Geometry check sheet. Reference: the model listing, model coordinates, mm. A direction names the side the tool comes from. Round coordinates to 2 decimals unless told otherwise and drop trailing zeros. Order: outer loops, then holes, each group sorted by start corner. A loop starts at its lowest first (then second) coordinate and runs counter-clockwise, first axis right, second up. Notation, with made-up numbers: (43, -4) - (81, -4) arc R14 ccw to (81, 6) - close; hole circle Ø6 at (-16, 6.25). An arc over 180 degrees is marked (long way). One line per question, with ' | ' between items. Start each with the question number.
Q1. Sectioned sample at C-C, the plane x = 0. Give the number of separate pieces and of enclosed holes in the cut face, then the cut area to 3 significant figures.
Q2. Sectioned sample at A-A, the plane x = -30.5. Enter the section's corners in (y, z), then the cut area to 3 significant figures.
Q3. Material ranges on line 1 along Z through (x, y) = (9, 5); line 2 along Z through (x, y) = (-7, 34); line 3 along Y through (x, z) = (-33, -41.5), recorded low to high.
Q4. Gauge pin test, flat ends, axial feed: P1, Ø2, axis at x = -19.5, y = -16, coming from the +Z side; P2, Ø2, axis at y = -15.5, z = -18, coming from the +X side; P3, Ø5, axis at x = 23, y = 26.5, coming from the +Z side; P4, Ø1.5, axis at x = -31.5, z = -38.5, coming from the +Y side. Record the tip position at first contact, or that the pin passes through.
Q5. Sectioned sample at D-D, the plane y = -33. Enter the section's corners in (x, z), then the cut area to 3 significant figures.
Q6. Tool access check on faces 5 (the face through (-7.91, -10.316, -10.028)), 6 (the face through (-8, 7, -4)), 7 (the face through (-3.1, -3.1, -20)). Record the directions out of +Z, -Z, +X, -X, +Y, -Y that give a thin tool (end or side, any length) a straight path to the whole face; none if there is none.
Q7. Mould release check, pull along Y, two halves, no side actions. Record for faces 1 (the face through (-2.83, 3.087, -10.633)), 2 (the face through (-7.509, 23.846, -32.161)), 3 (the face through (-30, -3, -42)), 4 (the face through (-18, -10, -46)): +Y half, -Y half, draft (parallel to the pull), parting line (faces both ways), or undercut.
Q8. Sectioned sample at B-B, the plane z = -33.5. Enter the section's corners in (x, y), then the cut area to 3 significant figures.
Autodesk Inventor part; units mm, degrees
ref_plane "YZ Plane" through (0, 0, 0) normal (1, 0, 0) x (0, 1, 0)
ref_plane "XZ Plane" through (0, 0, 0) normal (0, 1, 0) x (-1, 0, 0)
ref_plane "XY Plane" through (0, 0, 0) normal (0, 0, 1) x (1, 0, 0)
sketch "草图1" plane through (0, 0, 0) normal (1, 0, 0) x (0, 1, 0)
  line L0 (0, 0) -> (13, 0)
  line L1 (13, 0) -> (13, -4)
  line L2 (13, -4) -> (10, -4)
  line L3 (10, -4) -> (10, -8)
  line L4 (10, -8) -> (13, -8)
  line L5 (13, -8) -> (13, -12)
  line L6 (13, -12) -> (18, -12)
  line L7 (18, -12) -> (18, -15)
  line L8 (0, 0) -> (0, -15)
  line L9 (18, -15) -> (25, -15)
  line L10 (0, 0) -> (0, -46)
  line L11 (0, -46) -> (41, -46)
  line L12 (41, -46) -> (41, -40)
  line L13 (41, -40) -> (25, -40)
  line L14 (25, -40) -> (25, -15)
  dimension "d0" = 13
  dimension "d1" = 4
  dimension "d2" = 3
  dimension "d3" = 4
  dimension "d4" = 3
  dimension "d5" = 4
  dimension "d6" = 5
  dimension "d7" = 3
  dimension "d8" = 25
  dimension "d9" = 46
  dimension "d10" = 41
  dimension "d11" = 6
  dimension "d12" = 16
revolve "旋转1" add sketch "草图1" angle 360 about axis through (0, 0, 0) along (0, 0, -1)
sketch "草图2" plane through (0, 0, 0) normal (0, 0, 1) x (1, 0, 0)
  circle A0 centre (0, 0) radius 13
hole "孔1" at (0, 0, 0) direction (0, 0, -1) diameter 8.376 end through all
sketch "草图3" plane through (0, 0, -46) normal (0, 0, -1) x (-1, 0, 0)
  circle A0 centre (0, 0) radius 4.188
  circle A1 centre (0, 0) radius 41
  circle A2 centre (0, 0) radius 20
  dimension "d21" = 40
extrude "拉伸1" cut sketch "草图3" against normal blind 26 contours A2
fillet "圆角1" radius 5 1 edges at (20, 0, -20)
fillet "圆角2" radius 10 1 edges at (0, -25, -15)
sketch "草图4" plane through (0, 0, -40) normal (0, 0, 1) x (1, 0, 0)
  circle A0 centre (0, 0) radius 41
  circle A1 centre (0, 0) radius 33
  point P0 (-33, 0)
  dimension "d26" = 66
hole "孔2" at (-33, 0, -40) direction (0, 0, -1) diameter 7 end through all
sketch "草图5" plane through (0, 0, -40) normal (0, 0, 1) x (1, 0, 0)
  circle A0 centre (-33, 0) radius 3.5
  point P0 (0, 0)
hole "孔3" at (-33, 0, -40) direction (0, 0, -1) diameter 12 depth 2
pattern_circular "环形阵列1" count 4 over 360 about axis through (0, 0, -124.7558) along (0, 0, 1) of "孔3", "孔2"
chamfer "倒角1" distance 1 angle 45 1 edges at (0, 4.188, 0)
properties material "灰口铁"
Determined:
1) separate pieces: 4 | enclosed holes: 0 | area: 801 mm2
2) outline: (-27.4, -46) - (-2.45, -46) - (-2.45, -42) - (-5.45, -42) - (-5.45, -40) - (-27.4, -40) - close; (2.45, -46) - (27.4, -46) - (27.4, -40) - (5.45, -40) - (5.45, -42) - (2.45, -42) - close | area: 287 mm2
3) line 1: z = -20 to -8, -4 to 0 | line 2: z = -46 to -40 | line 3: y = -24.33 to -6, 6 to 24.33
4) P1: stops at z = -20.68 | P2: stops at x = 17.77 | P3: stops at z = -40 | P4: passes through
5) outline: (-24.33, -46) - (-3.5, -46) - (-3.5, -42) - (-6, -42) - (-6, -40) - (-24.33, -40) - close; (3.5, -46) - (24.33, -46) - (24.33, -40) - (6, -40) - (6, -42) - (3.5, -42) - close | area: 240 mm2
6) face 5: +Z | face 6: none | face 7: -Z
7) face 1: undercut | face 2: parting line | face 3: undercut | face 4: draft
8) outline: circle Ø50 at (0, 0); hole circle Ø40 at (0, 0) | area: 707 mm2
